from build123d import *

# Parameters (mm, degrees)
F0_R     = 38.1
F1_DEPTH = 9.525
F2_R     = 33.02
F3_DEPTH = 1.5875
F4_R     = 33.02
F5_DEPTH = 1.5875
F6_R     = 12.7
F6_R_2   = 1.27
F7_DEPTH = 25.4


with BuildPart() as f1:
    # F0 (on Top) → F1 (new body)
    with BuildSketch(Plane.XY):
        Circle(F0_R)
    extrude(amount=F1_DEPTH)

    # F2 (on face) → F3 (cut)
    with BuildSketch(Plane(origin=(0, 0, 0), x_dir=(1, 0, 0), z_dir=(0, 0, -1))):
        Circle(F2_R)
    extrude(amount=-F3_DEPTH, mode=Mode.SUBTRACT)

    # F4 (on face) → F5 (cut)
    with BuildSketch(Plane.XY.offset(9.525)):
        Circle(F4_R)
    extrude(amount=-F5_DEPTH, mode=Mode.SUBTRACT)

    # F6 (on face) → F7 (cut)
    with BuildSketch(Plane(origin=(0, 0, 1.5875), x_dir=(1, 0, 0), z_dir=(0, 0, -1))):
        Circle(F6_R)
        with Locations((-19.05, 0)):
            Circle(F6_R_2)
        with Locations((-13.470384, -13.470384)):
            Circle(F6_R_2)
        with Locations((0, -19.05)):
            Circle(F6_R_2)
        with Locations((13.470384, -13.470384)):
            Circle(F6_R_2)
        with Locations((19.05, 0)):
            Circle(F6_R_2)
        with Locations((13.470384, 13.470384)):
            Circle(F6_R_2)
        with Locations((0, 19.05)):
            Circle(F6_R_2)
        with Locations((-13.470384, 13.470384)):
            Circle(F6_R_2)
    extrude(amount=-F7_DEPTH, mode=Mode.SUBTRACT)


solid = f1.part
Work out the finished part from the listing and answer in its coordinate system (mm). A direction names the side the tool comes from. Coordinates: 2 decimals unless noted, no trailing zeros. Loops run counter-clockwise (first coordinate to the right, second up) from the corner with the lowest first, then second, coordinate; pieces in that order, holes last. Notation, with made-up numbers: (-38, 6) -> (-19, 6) arc R24 ccw to (-19, 45) -> close; hole circle Ø9 at (87, 31.25). An arc over 180 degrees is marked (long way). Answer as CSV lines item,"result".
1) The part is cut by section B-B (y = 10). Give the vertices of the cut face in (x, z) (1 decimal), and give its area (3 significant figures).
A:
outline,"(-36.8, 0) -> (-31.5, 0) -> (-31.5, 1.6) -> (-7.8, 1.6) -> (-7.8, 7.9) -> (-31.5, 7.9) -> (-31.5, 9.5) -> (-36.8, 9.5) -> close; (7.8, 1.6) -> (31.5, 1.6) -> (31.5, 0) -> (36.8, 0) -> (36.8, 9.5) -> (31.5, 9.5) -> (31.5, 7.9) -> (7.8, 7.9) -> close"
area,"401 mm²"
2) Flat-ended cylindrical pins translate along their axes: pin 1 (20 mm diameter, centred on x = 15.5, y = -6.5, fed in from -Z); pin 2 (1 mm diameter, centred on x = 3, z = 8, fed in from +Y); pin 3 (3.5 mm diameter, centred on x = -13.47, y = -13.47, fed in from +Z). Find the tip coordinate at first contact, or state that the pin passes through.
A:
pin 1,"stops at z = 1.59"
pin 2,"stops at y = 38.02"
pin 3,"stops at z = 7.94"
3) For faces 4 (the face through (31.5, 9.9, 8.7)), 5 (the face through (-11.5, 31.2, 0)), 6 (the face through (0, 14, 1.588)), determine the directions among +Z, -Z, +X, -X, +Y, -Y from which every point of the face is accessible in a straight line to the end or side of a thin tool.
A:
face 4,"+Z"
face 5,"-Z, +X, -X, +Y, -Y"
face 6,"-Z"
4) For a pull along Y with two mould halves and no side action, classify faces 1 (the face through (-30.235, -23.183, 4.696)), 2 (the face through (31.5, -9.9, 0.8)), 3 (the face through (-11.5, 31.2, 9.525)) as released by +Y, released by -Y, zero draft, split by the parting line, or undercut.
A:
face 1,"split by the parting line"
face 2,"undercut"
face 3,"zero draft"
5) The part is cut by section C-C (x = -19.05). Give the vertices of the cut face in (y, z) (1 decimal), and give its area (3 significant figures).
A:
outline,"(-33, 0) -> (-27, 0) -> (-27, 1.6) -> (-1.3, 1.6) -> (-1.3, 7.9) -> (-27, 7.9) -> (-27, 9.5) -> (-33, 9.5) -> close; (1.3, 1.6) -> (27, 1.6) -> (27, 0) -> (33, 0) -> (33, 9.5) -> (27, 9.5) -> (27, 7.9) -> (1.3, 7.9) -> close"
area,"441 mm²"
6) The part is cut by section A-A (x = 0). Give the vertices of the cut face in (y, z) (1 decimal), and give its area (3 significant figures).
A:
outline,"(-38.1, 0) -> (-33, 0) -> (-33, 1.6) -> (-20.3, 1.6) -> (-20.3, 7.9) -> (-33, 7.9) -> (-33, 9.5) -> (-38.1, 9.5) -> close; (-17.8, 1.6) -> (-12.7, 1.6) -> (-12.7, 7.9) -> (-17.8, 7.9) -> close; (12.7, 1.6) -> (17.8, 1.6) -> (17.8, 7.9) -> (12.7, 7.9) -> close; (20.3, 1.6) -> (33, 1.6) -> (33, 0) -> (38.1, 0) -> (38.1, 9.5) -> (33, 9.5) -> (33, 7.9) -> (20.3, 7.9) -> close"
area,"323 mm²"
7) Straight lines are drawn through the part: probe 1 along X at (y, z) = (13, 2); probe 2 along Z at (x, y) = (21, -10.5); probe 3 along X at (y, z) = (12, 1). For each, find the intervals that lie inside material, in ascending order.
A:
probe 1,"x = -35.81 to -14.65, -12.29 to 12.29, 14.65 to 35.81"
probe 2,"z = 1.59 to 7.94"
probe 3,"x = -36.16 to -30.76, 30.76 to 36.16"
